Check sheet for the modelled part. Datum: model origin and axes. Units: mm. A direction names the side the tool comes from. Round coordinates to 2 decimals unless told otherwise and drop trailing zeros. Write each loop counter-clockwise with the first axis right and the second up, starting at its lowest first coordinate (ties: lowest second). Pieces come first, ordered by that corner, then holes. Notation, with made-up numbers: (8, -19) - (20, -19) arc R18 ccw to (20, -11) - close; hole circle Ø10 at (41, -15.75). An arc over 180 degrees is marked (long way). Use one line per item in the form item = value. Start each with the question number.
1) Section check B-B (x = -12.5). Record the boundary of the cut face in (y, z), then the cut area to 3 significant figures.
2) Section check D-D (y = 8). Record the boundary of the cut face in (x, z), then the cut area to 3 significant figures.
3) Set-up check for faces 5 (the face through (0, 15, 2.308)), 6 (the face through (12.95, 0.99, 1.43)): record each of +Z, -Z, +X, -X, +Y, -Y from which the full face is reachable in a straight line by a thin tool's end or side.
4) Section check C-C (z = 12.5). Record the boundary of the cut face in (x, y).
5) Scan lines: probe 1 along X at (y, z) = (0.65, 0); probe 2 along Y at (x, z) = (-9, 11.5); probe 3 along X at (y, z) = (0.7, 12.5). Record each from-to range of solid material in increasing order.
6) Gauge pin test, flat ends, axial feed: P1, Ø1.5, axis at x = 11, z = -7.5, coming from the +Y side; P2, Ø6, axis at y = 11, z = 2, coming from the -X side; P3, Ø2, axis at y = 15.5, z = -2.5, coming from the -X side. Record the tip position at first contact, or that the pin passes through.
7) Section check A-A (x = 0). Record the boundary of the cut face in (y, z).
8) Draft check along X on faces 1 (the face through (0, 1, -14)), 2 (the face through (-4, 2, 0)), 3 (the face through (-10.648, 0.986, -13.887)), 4 (the face through (0, 1, 11)). Enter one of: +X half, -X half, draft (parallel to the pull), parting line (faces both ways), or undercut.
from build123d import *

# Parameters (mm, degrees)
SKETCH_1_R      = 17.5
SKETCH_1_R_2    = 1.5
EXTRUDE_1_DEPTH = 2
EXTRUDE_2_DEPTH = 25
SKETCH_3_R      = 3
EXTRUDE_3_DEPTH = 2


with BuildPart() as part:
    # 草图1 → 凸台-拉伸1 (new body)
    with BuildSketch(Plane(origin=(0, 0, 0), x_dir=(1, 0, 0), z_dir=(0, 1, 0))):
        with Locations(Location((0, 0, 0), (0, 0, 270))):
            Circle(SKETCH_1_R)
        with Locations(Location((0, 12.5, 0), (0, 0, 270))):
            Circle(SKETCH_1_R_2, mode=Mode.SUBTRACT)
        with Locations(Location((12.5, 0, 0), (0, 0, 270))):
            Circle(SKETCH_1_R_2, mode=Mode.SUBTRACT)
        with Locations(Location((0, -12.5, 0), (0, 0, 270))):
            Circle(SKETCH_1_R_2, mode=Mode.SUBTRACT)
        with Locations(Location((-12.5, 0, 0), (0, 0, 270))):
            Circle(SKETCH_1_R_2, mode=Mode.SUBTRACT)
    extrude(amount=EXTRUDE_1_DEPTH)

    # 草图2 → 凸台-拉伸2 (add)
    with BuildSketch(Plane(origin=(0, 2, 0), x_dir=(1, 0, 0), z_dir=(0, 1, 0))):
        with BuildLine():
            Line((-1.916694525, -2.307873934), (1.916694525, -2.307873934))
            ThreePointArc((1.916694525, -2.307873934), (0, 3), (-1.916694525, -2.307873934))
        make_face()
    extrude(amount=EXTRUDE_2_DEPTH)

    # 草图3 → 凸台-拉伸3 (add)
    with BuildSketch(Plane(origin=(0, 2, 0), x_dir=(1, 0, 0), z_dir=(0, 1, 0))):
        with Locations(Location((0, 0, 0), (0, 0, 309.709708175))):
            Circle(SKETCH_3_R)
    extrude(amount=EXTRUDE_3_DEPTH)


solid = part.part
Results are:
q1.outline = (0, -12.25) - (2, -12.25) - (2, -1.5) - (0, -1.5) - close; (0, 1.5) - (2, 1.5) - (2, 12.25) - (0, 12.25) - close
q1.area = 43.0 mm²
q2.outline = (-1.92, 2.31) arc R3 ccw (long way) to (1.92, 2.31) - close
q2.area = 26.5 mm²
q3.face_5 = +Z, +X, -X, +Y
q3.face_6 = +Y, -Y
q4.outline = (-12.25, 0) - (-1.5, 0) - (-1.5, 2) - (-12.25, 2) - close; (1.5, 0) - (12.25, 0) - (12.25, 2) - (1.5, 2) - close
q5.probe_1 = -17.5 to -14, -11 to 11, 14 to 17.5
q5.probe_2 = 0 to 2
q5.probe_3 = -12.25 to -1.5, 1.5 to 12.25
q6.P1 = 2
q6.P2 = -3
q6.P3 = -2.6
q7.outline = (0, -17.5) - (2, -17.5) - (2, -14) - (0, -14) - close; (0, -11) - (2, -11) - (2, -3) - (27, -3) - (27, 2.31) - (4, 2.31) - (4, 3) - (2, 3) - (2, 11) - (0, 11) - close; (0, 14) - (2, 14) - (2, 17.5) - (0, 17.5) - close
q8.face_1 = undercut
q8.face_2 = draft
q8.face_3 = parting line
q8.face_4 = undercut
